Here's how the part is built. I have some questions about the finished solid (model axes, mm). A direction names the side the tool comes from. Give positions to 0.01 mm unless a question says otherwise; leave off trailing zeros. Order: outer loops, then holes, each group sorted by start corner. A loop starts at its lowest first (then second) coordinate and runs counter-clockwise, first axis right, second up. Notation, with made-up numbers: (67.25, 87) - (116.25, 87) arc R25 ccw to (116.25, 111) - close; hole circle Ø4 at (58.25, 82.5). An arc over 180 degrees is marked (long way). One line per question, with ' | ' between items.
Solid Edge part; units mm, degrees
sketch "Sketch1" plane through (0, 0, 0) normal (1, 0, 0) x (0, 1, 0)
  line L0 (0, 25) -> (102.846, 147.5671)
  line L1 (102.846, 147.5671) -> (122.846, 147.5671)
  line L2 (122.846, 147.5671) -> (122.846, 0)
  line L3 (122.846, 0) -> (5.5389, 0)
  line L4 (5.5389, 0) -> (0, 0)
  line L5 (0, 0) -> (0, 25)
extrude "Protrusion1" add sketch "Sketch1" against normal blind 190
sketch "Sketch2" plane through (-95, 112.846, 147.5671) normal (0, 0, 1) x (1, 0, 0)
  line L0 (88, -10) -> (88, -105.85)
  line L1 (88, -105.85) -> (-86, -105.85)
  line L2 (-86, -105.85) -> (-86, -10)
  line L3 (-86, -10) -> (0, -10)
  line L4 (0, -10) -> (88, -10)
extrude "Cutout1" cut sketch "Sketch2" against normal blind 140.57
sketch "Sketch3" plane through (-95, 61.423, 0) normal (0, 0, -1) x (0, 1, 0)
  line L0 (-2.2305, 50) -> (-2.2305, -50)
  line L1 (-2.2305, -50) -> (7.7695, -50)
  line L2 (7.7695, -50) -> (7.7695, 50)
  line L3 (7.7695, 50) -> (-2.2305, 50)
extrude "VaciadoExtruido_3" cut sketch "Sketch3" against normal blind 7
sketch "Sketch4" plane through (-95, 51.423, 86.2836) normal (0, -0.766, 0.6428) x (1, 0, 0)
  circle A0 centre (91.5, 70) radius 1.75
extrude "Cutout2" cut sketch "Sketch4" against normal blind 30
sketch "Sketch5" plane through (-95, 51.423, 86.2836) normal (0, -0.766, 0.6428) x (1, 0, 0)
  circle A0 centre (91.5, -70) radius 1.75
extrude "VaciadoExtruido_14" cut sketch "Sketch5" against normal blind 30
sketch "Sketch6" plane through (-95, 51.423, 86.2836) normal (0, -0.766, 0.6428) x (1, 0, 0)
  circle A0 centre (-90.5, 70) radius 1.75
extrude "VaciadoExtruido_15" cut sketch "Sketch6" against normal blind 30
sketch "Sketch7" plane through (-95, 51.423, 86.2836) normal (0, -0.766, 0.6428) x (1, 0, 0)
  circle A0 centre (-90.5, -70) radius 1.75
extrude "VaciadoExtruido_16" cut sketch "Sketch7" against normal blind 30
1) I want a section at D-D (z = 125.5). State how many separate pieces and enclosed holes the cut face has, plus the area to 3 significant figures.
Model answer:
separate pieces: 1 | enclosed holes: 2 | area: 4,070 mm2
2) On a 3-axis mill with a long thin cutter (end or side, diameter ignored), from which of +Z, -Z, +X, -X, +Y, -Y can I reach the whole of each face in a straight line? I mean faces 1 (the face through (-94, 113, 147.567)), 2 (the face through (-95, 102.846, 78)), 3 (the face through (-45, 64, 3)). Say none if no direction works.
Model answer:
face 1: +Z, +X, -X, +Y, -Y | face 2: +Z | face 3: +Z, -Z
3) I'm going to push flat-ended pins straight in: P1, Ø8, axis at x = -105.5, z = 62.5, coming from the -Y side; P2, Ø1, axis at x = -46, y = 92, coming from the +Z side. Where does each tip first touch, or does it pass through?
Model answer:
P1: stops at y = 102.85 | P2: stops at z = 7
4) I want a section at A-A (x = -76.5). List the corners of the cut face in (y, z) for me.
Model answer:
outline: (0, 0) - (59.19, 0) - (59.19, 7) - (7, 7) - (7, 33.34) - (0, 25) - close; (69.19, 0) - (122.85, 0) - (122.85, 147.57) - (102.85, 147.57) - (102.85, 7) - (69.19, 7) - close
5) Thinking about a two-plate mould opening in X: for faces 4 (the face through (-94, 122.846, 75)), 5 (the face through (-181, 65, 63)), 6 (the face through (-190, 74, 58)), which applies, +X half, -X half, draft (parallel to the pull), parting line (faces both ways), or undercut?
Model answer:
face 4: draft | face 5: undercut | face 6: -X half
6) I want a section at B-B (x = -148.5). List the corners of the cut face in (y, z) for me, plus the area to 3 significant figures.
Model answer:
outline: (0, 0) - (122.85, 0) - (122.85, 147.57) - (102.85, 147.57) - (102.85, 7) - (7, 7) - (7, 33.34) - (0, 25) - close | area: 3,830 mm2
7) Please list where these lines run through material, in increasing order: L1, parallel to X at y = 17, z = 7.5; L2, parallel to Y at x = -169.5, z = 11.5; L3, parallel to Z at x = -125, y = 89.
Model answer:
L1: x = -190 to -181, -7 to 0 | L2: y = 0 to 7, 102.85 to 122.85 | L3: z = 0 to 7
8) I want a section at C-C (z = 67). List the corners of the cut face in (x, y) for me.
Model answer:
outline: (-190, 35.24) - (-181, 35.24) - (-181, 102.85) - (-7, 102.85) - (-7, 35.24) - (0, 35.24) - (0, 122.85) - (-190, 122.85) - close
